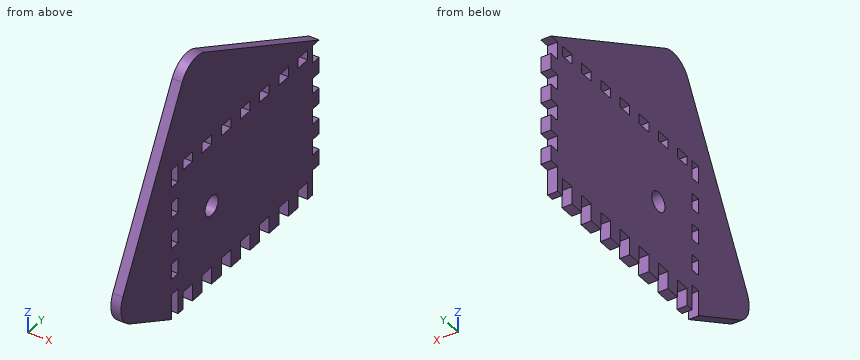
```python
from build123d import *

# Parameters (mm, degrees)
SCHIZZO1_W                   = 50
SCHIZZO1_H                   = 80
ESTRUSIONE_ESTRUSIONE1_DEPTH = 4
SCHIZZO2_W                   = 4
SCHIZZO2_H                   = 2.857142857
SCHIZZO2_W_2                 = 7
ESTRUSIONE_ESTRUSIONE2_DEPTH = 4
SCHIZZO3_W                   = 4
SCHIZZO3_H                   = 5.714285715
SCHIZZO3_W_2                 = 7
ESTRUSIONE_ESTRUSIONE3_DEPTH = 4
RIPETIZIONE_A_L1_COUNT       = 6
RIPETIZIONE_A_L1_PITCH       = 11.428571
SCHIZZO4_W                   = 6.25
SCHIZZO4_H                   = 4
ESTRUSIONE_ESTRUSIONE4_DEPTH = 4
RIPETIZIONE_A_L2_COUNT       = 4
RIPETIZIONE_A_L2_PITCH       = 12.5
ESTRUSIONE_ESTRUSIONE5_DEPTH = 4
RACCORDO1_R                  = 10
SCHIZZO6_R                   = 3.9
TAGLIO_ESTRUSIONE1_DEPTH     = 4


with BuildPart() as part:
    # Schizzo1 → Estrusione-Estrusione1 (new body)
    with BuildSketch(Plane(origin=(0, 0, 0), x_dir=(0, 0, -1), z_dir=(1, 0, 0))):
        with Locations((25, 40)):
            Rectangle(SCHIZZO1_W, SCHIZZO1_H)
    extrude(amount=ESTRUSIONE_ESTRUSIONE1_DEPTH)

    # Schizzo2 → Estrusione-Estrusione2 (add)
    with BuildSketch(Plane(origin=(4, 0, 0), x_dir=(0, 0, -1), z_dir=(1, 0, 0))):
        with Locations((-2, 78.571428572)):
            Rectangle(SCHIZZO2_W, SCHIZZO2_H)
        with Locations((53.5, 78.571428572)):
            Rectangle(SCHIZZO2_W_2, SCHIZZO2_H)
        with Locations((53.5, 1.428571429)):
            Rectangle(SCHIZZO2_W_2, SCHIZZO2_H)
        with Locations((-2, 1.428571429)):
            Rectangle(SCHIZZO2_W, SCHIZZO2_H)
    extrude(amount=-ESTRUSIONE_ESTRUSIONE2_DEPTH)

    # Schizzo3 → Estrusione-Estrusione3 (add)
    with BuildSketch(Plane(origin=(4, 0, 0), x_dir=(0, 0, -1), z_dir=(1, 0, 0))):
        with Locations((-2, 68.571428572)):
            Rectangle(SCHIZZO3_W, SCHIZZO3_H)
        with Locations((53.5, 68.571428572)):
            Rectangle(SCHIZZO3_W_2, SCHIZZO3_H)
    estrusione_estrusione3 = extrude(amount=-ESTRUSIONE_ESTRUSIONE3_DEPTH)

    # Ripetizione a L1: Estrusione-Estrusione3 ×6
    with Locations(*[(0, -i * RIPETIZIONE_A_L1_PITCH, 0) for i in range(1, RIPETIZIONE_A_L1_COUNT)]):
        add(estrusione_estrusione3)

    # Schizzo4 → Estrusione-Estrusione4 (add)
    with BuildSketch(Plane(origin=(4, 0, 0), x_dir=(0, 0, -1), z_dir=(1, 0, 0))):
        with Locations((6.25, 82)):
            Rectangle(SCHIZZO4_W, SCHIZZO4_H)
        with Locations((6.25, -2)):
            Rectangle(SCHIZZO4_W, SCHIZZO4_H)
    estrusione_estrusione4 = extrude(amount=-ESTRUSIONE_ESTRUSIONE4_DEPTH)

    # Ripetizione a L2: Estrusione-Estrusione4 ×4
    with Locations(*[(0, 0, -i * RIPETIZIONE_A_L2_PITCH) for i in range(1, RIPETIZIONE_A_L2_COUNT)]):
        add(estrusione_estrusione4)

    # Schizzo5 → Estrusione-Estrusione5 (add)
    with BuildSketch(Plane(origin=(4, 0, 0), x_dir=(0, 0, -1), z_dir=(1, 0, 0))):
        Polygon((46.875, -4), (57, -4), (39.160080614, -37.552008529), (-44.872956134, 7.129149682), (-4, 84), (-4, 80), (-4, -4), align=None)
    extrude(amount=-ESTRUSIONE_ESTRUSIONE5_DEPTH)

    # Raccordo1
    raccordo1_edges = [part.edges().sort_by_distance(p)[0] for p in [
        (2, -37.552008529, -39.160080614),
        (2, 7.129149682, 44.872956134),
    ]]
    fillet(raccordo1_edges, radius=RACCORDO1_R)

    # Schizzo6 → Taglio-Estrusione1 (cut)
    with BuildSketch(Plane(origin=(4, 0, 0), x_dir=(0, 0, -1), z_dir=(1, 0, 0))):
        with Locations((25, 20)):
            Circle(SCHIZZO6_R)
    extrude(amount=-TAGLIO_ESTRUSIONE1_DEPTH, mode=Mode.SUBTRACT)


solid = part.part
```
Design review of the part built by this model. Coordinates are the model's own, in mm. Coordinates: 2 decimals unless noted, no trailing zeros. Order: outer loops, then holes, each group sorted by start corner. A loop starts at its lowest first (then second) coordinate and runs counter-clockwise, first axis right, second up. Notation, with made-up numbers: (-9, -23) -> (46, -23) arc R30 cw to (46, 6) -> close; hole circle Ø9 at (80, 12.25). An arc over 180 degrees is marked (long way). One line per item, written item: value. Start each with the question number.
Q1. Take a section at B-B, the plane y = 63. State the section outline as (x, z) points, then the cut area to 3 significant figures.
Q2. Take a section at D-D, the plane z = 33.5. State the section outline as (x, y) points, then the cut area to 3 significant figures.
Q3. Take a section at A-A, the plane z = -25. State the section outline as (x, y) points, then the cut area to 3 significant figures.
Q4. Insertion check: pin 1 Ø2 at (x, y) = (3, 73.5) entering from -Z; pin 2 Ø1.2 at (x, z) = (2.5, -55) entering from -Y; pin 3 Ø2 at (x, z) = (2, -23) entering from -Y. Each pin has a flat end and moves straight along its axis. Give the tip position at first contact, or say it passes through.
Q5. For probe 1 along Y at (x, z) = (1.35, -25); probe 2 along Y at (x, z) = (1.05, -24.5); probe 3 along Y at (x, z) = (1.85, -0.5), list the stretches that pass through material, from the lowest coordinate up.
Q6. Take a section at C-C, the plane x = 2. Give the number of separate pieces and of enclosed holes in the cut face, then the cut area to 3 significant figures.
Values follow:
1. outline: (0, -50) -> (4, -50) -> (4, 0) -> (0, 0) -> close; (0, 4) -> (4, 4) -> (4, 15.17) -> (0, 15.17) -> close
1. area: 245 mm2
2. outline: (0, 1.08) -> (4, 1.08) -> (4, 28.52) -> (0, 28.52) -> close
2. area: 110 mm2
3. outline: (0, -30.02) -> (4, -30.02) -> (4, -4) -> (0, -4) -> close; (0, 0) -> (4, 0) -> (4, 16.1) -> (0, 16.1) -> close; (0, 23.9) -> (4, 23.9) -> (4, 80) -> (0, 80) -> close
3. area: 393 mm2
4. pin 1: stops at z = -50
4. pin 2: stops at y = -8.89
4. pin 3: stops at y = -29.49
5. probe 1: y = -30.02 to -4, 0 to 16.1, 23.9 to 80
5. probe 2: y = -29.76 to -4, 0 to 16.13, 23.87 to 80
5. probe 3: y = -17 to -4, 0 to 80
6. separate pieces: 1
6. enclosed holes: 12
6. area: 7,820 mm2
